```python
from build123d import *

# Parameters (mm, degrees)
SKETCH1_R               = 23.5
SKETCH1_R_2             = 3
BOSS_EXTRUDE1_DEPTH     = 4
SKETCH2_R               = 6
SKETCH2_R_2             = 3
BOSS_EXTRUDE2_DEPTH     = 16
SKETCH3_R               = 2.5
CUT_EXTRUDE1_DEPTH      = 21
SKETCH5_R               = 5.5
SKETCH5_R_2             = 3.5
CUT_EXTRUDE3_DEPTH      = 0.5
SKETCH6_R               = 5.5
SKETCH6_R_2             = 3.5
CUT_EXTRUDE4_DEPTH      = 0.5
SKETCH7_R               = 2
CUT_EXTRUDE5_DEPTH      = 10
CUT_EXTRUDE5_DEPTH_BACK = 10


with BuildPart() as part:
    # Sketch1 → Boss-Extrude1 (new body)
    with BuildSketch(Plane.XY):
        Circle(SKETCH1_R)
        Circle(SKETCH1_R_2, mode=Mode.SUBTRACT)
    extrude(amount=BOSS_EXTRUDE1_DEPTH)

    # Sketch2 → Boss-Extrude2 (add)
    with BuildSketch(Plane(origin=(0, 0, 0), x_dir=(-1, 0, 0), z_dir=(0, 0, -1))):
        Circle(SKETCH2_R)
        Circle(SKETCH2_R_2, mode=Mode.SUBTRACT)
    extrude(amount=BOSS_EXTRUDE2_DEPTH)

    # Sketch3 → Cut-Extrude1 (cut, through all)
    with BuildSketch(Plane.XY.offset(4)):
        with Locations((-17.5, 0)):
            Circle(SKETCH3_R)
        with Locations((-8.75, 15.155444566)):
            Circle(SKETCH3_R)
        with Locations((8.75, 15.155444566)):
            Circle(SKETCH3_R)
        with Locations((17.5, 0)):
            Circle(SKETCH3_R)
        with Locations((8.75, -15.155444566)):
            Circle(SKETCH3_R)
        with Locations((-8.75, -15.155444566)):
            Circle(SKETCH3_R)
    extrude(amount=-CUT_EXTRUDE1_DEPTH, mode=Mode.SUBTRACT)

    # Sketch5 → Cut-Extrude3 (cut)
    with BuildSketch(Plane.XY.offset(4)):
        Circle(SKETCH5_R)
        Circle(SKETCH5_R_2, mode=Mode.SUBTRACT)
    extrude(amount=-CUT_EXTRUDE3_DEPTH, mode=Mode.SUBTRACT)

    # Sketch6 → Cut-Extrude4 (cut)
    with BuildSketch(Plane(origin=(0, 0, -16), x_dir=(-1, 0, 0), z_dir=(0, 0, -1))):
        Circle(SKETCH6_R)
        Circle(SKETCH6_R_2, mode=Mode.SUBTRACT)
    extrude(amount=-CUT_EXTRUDE4_DEPTH, mode=Mode.SUBTRACT)

    # Sketch7 → Cut-Extrude5 (cut, two sides)
    with BuildSketch(Plane(origin=(0, 0, 0), x_dir=(1, 0, 0), z_dir=(0, 1, 0))) as cut_extrude5_sk:
        with Locations((0, 8)):
            Circle(SKETCH7_R)
    extrude(amount=CUT_EXTRUDE5_DEPTH, mode=Mode.SUBTRACT)
    extrude(cut_extrude5_sk.sketch, amount=-CUT_EXTRUDE5_DEPTH_BACK, mode=Mode.SUBTRACT)


solid = part.part
```
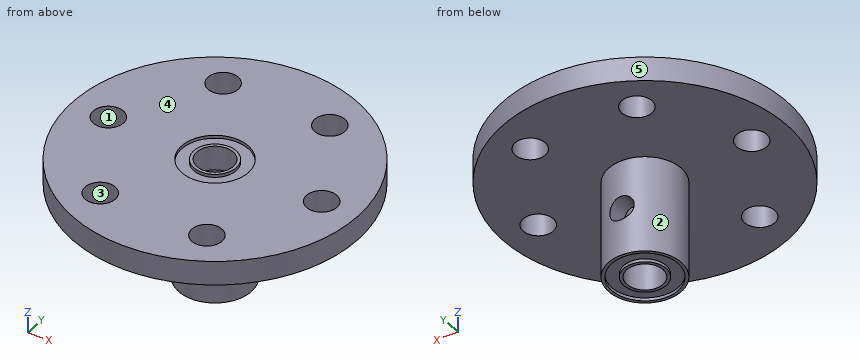
The model under review builds one solid part; all positions refer to its coordinate system, in mm. Face numbers are marked on the shaded views. A direction names the side the tool comes from. Give positions to 0.01 mm unless a question says otherwise; leave off trailing zeros. Write each loop counter-clockwise with the first axis right and the second up, starting at its lowest first coordinate (ties: lowest second). Pieces come first, ordered by that corner, then holes. Notation, with made-up numbers: M 42,60.5 L 82,60.5 A26 cw 82,92.5 Z; hole C 30,-32 d11. An arc over 180 degrees is marked long. Write each question's results on one line, items separated by ' | '. Start each with the question number.
1. We need section B-B (z = -8). Write out the cut boundary in (x, y), and give its area (3 significant figures).
2. For probe 1 along Y at (x, z) = (8.75, 2.3); probe 2 along Z at (x, y) = (0, 3.45); probe 3 along Y at (x, z) = (-6.5, 1.5), list the stretches that pass through material, from the lowest coordinate up. Write a range as [from, to].
3. For the marked faces 1 and 2, list the 3-axis set-ups (+Z, -Z, +X, -X, +Y, -Y) from which the entire face can be reached by the end or side of a thin tool; tool diameter is ignored.
4. We need section C-C (x = 17.5). Write out the cut boundary in (y, z), and give its area (3 significant figures).
5. We need section A-A (x = -7). Write out the cut boundary in (y, z).
6. Mouldability with a two-part tool opening along X and no side actions: class the marked faces 3, 4 and 5 as released by +X, released by -X, zero draft, split by the parting line, or undercut.
7. Insertion check: pin 1 Ø8 at (x, y) = (8.75, -15.16) entering from -Z; pin 2 Ø3 at (x, z) = (0, -8) entering from +Y; pin 3 Ø6.5 at (x, z) = (0, -8) entering from -Y; pin 4 Ø3 at (y, z) = (2.5, -6) entering from -X. Each pin has a flat end and moves straight along its axis. Give the tip position at first contact, or say it passes through.
8. We need section D-D (z = -1.5). Write out the cut boundary in (x, y), and give its area (3 significant figures).
Results found:
1) outline: M -2,-5.66 L -2,-2.24 A3 cw -2,2.24 L -2,5.66 A6 ccw Z; M 2,-5.66 A6 ccw 2,5.66 L 2,2.24 A3 cw 2,-2.24 Z | area: 59.8 mm^2
2) probe 1: y = [-21.81, -17.66], [-12.66, 12.66], [17.66, 21.81] | probe 2: z = [-16, -10], [-6, 4] | probe 3: y = [-22.58, -16.25], [-14.07, 14.07], [16.25, 22.58]
3) face 1: +Z, -Z | face 2: -Z
4) outline: M -15.68,0 L -2.5,0 L -2.5,4 L -15.68,4 Z; M 2.5,0 L 15.68,0 L 15.68,4 L 2.5,4 Z | area: 105 mm^2
5) outline: M -22.43,0 L -16.94,0 L -16.94,4 L -22.43,4 Z; M -13.37,0 L 13.37,0 L 13.37,4 L -13.37,4 Z; M 16.94,0 L 22.43,0 L 22.43,4 L 16.94,4 Z
6) face 3: undercut | face 4: zero draft | face 5: split by the parting line
7) pin 1: stops at z = 0 | pin 2: passes through | pin 3: stops at y = -6 | pin 4: stops at x = -5.92
8) outline: C 0,0 d12; hole C 0,0 d6 | area: 84.8 mm^2
